```python
from build123d import *

# Parameters (mm, degrees)
SKETCH1_R           = 50
BOSS_EXTRUDE1_DEPTH = 100
SKETCH3_R           = 5
BOSS_EXTRUDE3_DEPTH = 5
SKETCH4_R           = 5
BOSS_EXTRUDE4_DEPTH = 5
SKETCH5_R           = 30
CUT_EXTRUDE1_DEPTH  = 127.736251111


with BuildPart() as part:
    # Sketch1 → Boss-Extrude1 (new body)
    with BuildSketch(Plane.XY):
        with Locations((0.369408828, 0)):
            Circle(SKETCH1_R)
    extrude(amount=BOSS_EXTRUDE1_DEPTH)

    # Sketch3 → Boss-Extrude3 (add)
    with BuildSketch(Plane(origin=(0, 0, 0), x_dir=(-1, 0, 0), z_dir=(0, 0, -1))):
        with Locations(Location((0, 35, 0), (0, 0, 180))):
            Circle(SKETCH3_R)
        with Locations(Location((35, 0, 0), (0, 0, 180))):
            Circle(SKETCH3_R)
        with Locations(Location((0, -35, 0), (0, 0, 180))):
            Circle(SKETCH3_R)
        with Locations(Location((-35, 0, 0), (0, 0, 180))):
            Circle(SKETCH3_R)
    extrude(amount=BOSS_EXTRUDE3_DEPTH)

    # Sketch4 → Boss-Extrude4 (add)
    with BuildSketch(Plane.XY.offset(100)):
        with Locations((23.764833651, 32.175031958)):
            Circle(SKETCH4_R)
        with Locations((32.175031958, -23.764833651)):
            Circle(SKETCH4_R)
        with Locations((-23.764833651, -32.175031958)):
            Circle(SKETCH4_R)
        with Locations((-32.175031958, 23.764833651)):
            Circle(SKETCH4_R)
    extrude(amount=BOSS_EXTRUDE4_DEPTH)

    # Sketch5 → Cut-Extrude1 (cut, through all)
    with BuildSketch(Plane.XY.offset(100)):
        with Locations((-0.009474688, 0.189441758)):
            Circle(SKETCH5_R)
    extrude(amount=-CUT_EXTRUDE1_DEPTH, mode=Mode.SUBTRACT)


solid = part.part
```
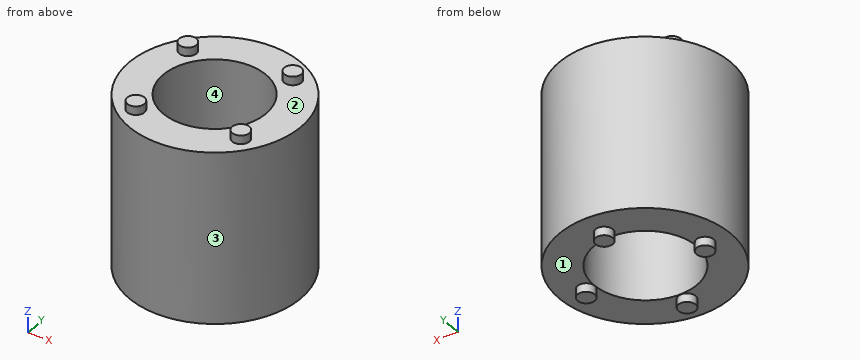
Here's how the part is built. I have some questions about the finished solid (model axes, mm). Face numbers are marked on the shaded views. A direction names the side the tool comes from. Coordinates: 2 decimals unless noted, no trailing zeros. Loops run counter-clockwise (first coordinate to the right, second up) from the corner with the lowest first, then second, coordinate; pieces in that order, holes last. Notation, with made-up numbers: (10, 85) - (62, 85) arc R26 ccw to (62, 102) - close; hole circle Ø6 at (60, 58). An arc over 180 degrees is marked (long way). Answer as CSV lines item,"result".
Q1. For the marked faces 1 and 2, which set-ups out of +Z, -Z, +X, -X, +Y, -Y let a thin tool reach every point of the face, with its end or its side?
Response:
face 1,"-Z"
face 2,"+Z"
Q2. For pin 1 (10 mm diameter, centred on x = 40, z = 16.5, fed in from -Y); pin 2 (1.5 mm diameter, centred on y = -1, z = 25, fed in from -X); pin 3 (12 mm diameter, centred on x = 27, y = 11, fed in from -Z); pin 4 (12 mm diameter, centred on y = -6, z = 15.5, fed in from +X), each with a flat end and sliding along its axis, tell me the tip position at first contact or that it passes through.
Response:
pin 1,"y = -36.07"
pin 2,"x = -49.63"
pin 3,"z = 0"
pin 4,"x = 50.37"
Q3. If we section it at D-D, the plane z = 55: Write out the boundary of the cut face in (x, y).
Response:
outline,"circle Ø100 at (0.37, 0); hole circle Ø60 at (-0.01, 0.19)"
Q4. If we section it at C-C, the plane x = 35: Write out the boundary of the cut face in (y, z), and give its area (3 significant figures).
Response:
outline,"(-36.07, 0) - (-5, 0) - (-5, -5) - (5, -5) - (5, 0) - (36.07, 0) - (36.07, 100) - (-19.64, 100) - (-19.64, 105) - (-27.89, 105) - (-27.89, 100) - (-36.07, 100) - close"
area,"7,300 mm2"
Q5. If I drill on L1, parallel to Z at x = 31, y = 30.5; L2, parallel to X at y = -18, z = 73.5; L3, parallel to X at y = -4.5, z = 86, over which ranges is the centre line in solid material (lowest first)? Write a range as [from, to].
Response:
L1,"[0, 100]"
L2,"[-46.28, -23.87], [23.85, 47.02]"
L3,"[-49.43, -29.64], [29.62, 50.17]"
Q6. We'd pull the mould along Y, two halves only. Please class the marked faces 3 and 4: pulls with the +Y half, pulls with the -Y half, needs draft (parallel to the pull), parting line crosses it, or undercut.
Response:
face 3,"parting line crosses it"
face 4,"undercut"
Q7. If we section it at A-A, the plane y = -13: Write out the boundary of the cut face in (x, z), and give its area (3 significant figures).
Response:
outline,"(-47.91, 0) - (-26.95, 0) - (-26.95, 100) - (-47.91, 100) - close; (26.94, 0) - (48.65, 0) - (48.65, 100) - (26.94, 100) - close"
area,"4,270 mm2"
Q8. If we section it at B-B, the plane x = -13: Write out the boundary of the cut face in (y, z), and give its area (3 significant figures).
Response:
outline,"(-48.18, 0) - (-26.85, 0) - (-26.85, 100) - (-48.18, 100) - close; (27.23, 0) - (48.18, 0) - (48.18, 100) - (27.23, 100) - close"
area,"4,230 mm2"
